from build123d import *

# Parameters (mm, degrees)
SKETCH1_W           = 38.09940225
SKETCH1_H           = 39.297540676
SKETCH1_R           = 3.7970867
BOSS_EXTRUDE1_DEPTH = 40
SKETCH1_3_R         = 3.7970867
CUT_EXTRUDE1_DEPTH  = 20


with BuildPart() as part:
    # Sketch1 → Boss-Extrude1 (new body)
    with BuildSketch(Plane.XY):
        with Locations((10.016557459, -10.016557459)):
            Rectangle(SKETCH1_W, SKETCH1_H)
        with Locations((10.016557459, -10.016557459)):
            Circle(SKETCH1_R, mode=Mode.SUBTRACT)
        with Locations((10.016557459, -10.016557459)):
            Circle(SKETCH1_R)
    extrude(amount=BOSS_EXTRUDE1_DEPTH)

    # Sketch1_3 → Cut-Extrude1 (cut)
    with BuildSketch(Plane.XY):
        with Locations((10.016557459, -10.016557459)):
            Circle(SKETCH1_3_R)
    extrude(amount=CUT_EXTRUDE1_DEPTH, mode=Mode.SUBTRACT)


solid = part.part
Verification items for the finished model (mm, model axes). Round coordinates to 2 decimals unless told otherwise and drop trailing zeros. Loops run counter-clockwise (first coordinate to the right, second up) from the corner with the lowest first, then second, coordinate; pieces in that order, holes last. Notation, with made-up numbers: (-1.5, -13) - (14.5, -13) arc R19 cw to (14.5, 15) - close; hole circle Ø1 at (23, 82). An arc over 180 degrees is marked (long way). Answer in a Markdown table with one row per item. Add a question column.
Q1. Section check A-A on x = 7. Enter the section's corners in (y, z), plus the area to 3 significant figures.
Q2. Section check B-B on y = -8. Enter the section's corners in (x, z).
Q3. Release check for a two-part mould opening along X. For faces 1 (the face through (13.524, -11.471, 9.86)), 2 (the face through (29.066, -10, 20)), 3 (the face through (10, -10, 40)), 4 (the face through (10, -10, 20)) record: pulls with the +X half, pulls with the -X half, needs draft (parallel to the pull), parting line crosses it, or undercut.
Q4. Material ranges on line 1 (Z direction, x = 8, y = -12); line 2 (Y direction, x = 12, z = 13.5); line 3 (X direction, y = -9, z = 15.5), recorded low to high.
Q5. Gauge pin test, flat end, axial feed: pin 1 (2.5 mm diameter, centred on x = 11.5, y = -11.5, fed in from -Z). Record the tip position at first contact, or that the pin passes through.
Q6. Section check C-C on z = 7. Enter the section's corners in (x, y), plus the area to 3 significant figures.
Found:
| question | item | result |
|---|---|---|
| 1 | outline | (-29.67, 0) - (-12.32, 0) - (-12.32, 20) - (-7.71, 20) - (-7.71, 0) - (9.63, 0) - (9.63, 40) - (-29.67, 40) - close |
| 1 | area | 1,480 mm² |
| 2 | outline | (-9.03, 0) - (6.8, 0) - (6.8, 20) - (13.23, 20) - (13.23, 0) - (29.07, 0) - (29.07, 40) - (-9.03, 40) - close |
| 3 | face 1 | undercut |
| 3 | face 2 | pulls with the +X half |
| 3 | face 3 | needs draft |
| 3 | face 4 | undercut |
| 4 | line 1 | z = 20 to 40 |
| 4 | line 2 | y = -29.67 to -13.25, -6.78 to 9.63 |
| 4 | line 3 | x = -9.03 to 6.36, 13.68 to 29.07 |
| 5 | pin 1 | stops at z = 20 |
| 6 | outline | (-9.03, -29.67) - (29.07, -29.67) - (29.07, 9.63) - (-9.03, 9.63) - close; hole circle Ø7.59 at (10.02, -10.02) |
| 6 | area | 1,450 mm² |
